Verification items for the finished model (mm, model axes). A direction names the side the tool comes from. Coordinates: 2 decimals unless noted, no trailing zeros. Order: outer loops, then holes, each group sorted by start corner. A loop starts at its lowest first (then second) coordinate and runs counter-clockwise, first axis right, second up. Notation, with made-up numbers: M 13,86.25 L 36,86.25 A31 ccw 36,112.25 Z; hole C 87.5,51 d7. An arc over 180 degrees is marked long. Use one line per item in the form item = value. Start each with the question number.
```python
from build123d import *

# Parameters (mm, degrees)
SKETCH1_R        = 3.175
EXTRUSION1_DEPTH = 6.35


with BuildPart() as part:
    # Sketch1 → Extrusion1 (new body)
    with BuildSketch(Plane.XY):
        with BuildLine():
            Line((-76.2, -6.35), (0, -6.35))
            ThreePointArc((0, -6.35), (6.35, 0), (0, 6.35))
            Line((0, 6.35), (-76.2, 6.35))
            ThreePointArc((-76.2, 6.35), (-82.55, 0), (-76.2, -6.35))
        make_face()
        with Locations((-76.2, 0)):
            Circle(SKETCH1_R, mode=Mode.SUBTRACT)
        with BuildLine():
            ThreePointArc((2.004434618, -2.462288948), (3.126764616, -0.551332964), (2.725704838, 1.62823774))
            Line((2.725704838, 1.62823774), (3.671276413, 2.755126062))
            Line((3.671276413, 2.755126062), (2.87351773, 3.424525079))
            Line((2.87351773, 3.424525079), (2.075759047, 4.093924095))
            Line((2.075759047, 4.093924095), (1.130187472, 2.967035773))
            ThreePointArc((1.130187472, 2.967035773), (-1.085913955, 2.983524071), (-2.772947665, 1.546410763))
            Line((-2.772947665, 1.546410763), (-4.221647367, 1.801855607))
            Line((-4.221647367, 1.801855607), (-4.402484579, 0.776276813))
            Line((-4.402484579, 0.776276813), (-4.583321791, -0.249301981))
            Line((-4.583321791, -0.249301981), (-3.134622089, -0.504746825))
            ThreePointArc((-3.134622089, -0.504746825), (-2.040850661, -2.432191107), (0.047242827, -3.174648503))
            Line((0.047242827, -3.174648503), (0.550370953, -4.556981669))
            Line((0.550370953, -4.556981669), (1.528966849, -4.200801892))
            Line((1.528966849, -4.200801892), (2.507562744, -3.844622115))
            Line((2.507562744, -3.844622115), (2.004434618, -2.462288948))
        make_face(mode=Mode.SUBTRACT)
    extrude(amount=EXTRUSION1_DEPTH)


solid = part.part
```
1. Material ranges on line 1 along X through (y, z) = (-2.75, 5.5); line 2 along Y through (x, z) = (-76.2, 4.25) (3 decimals); line 3 along X through (y, z) = (2, 4), recorded low to high.
2. Release check for a two-part mould opening along X. For faces 1 (the cylindrical face through (-82.55, 0.14, 3.13)), 2 (the flat face through (0.295, -3.856, 3.131)), 3 (the cylindrical face through (6.35, -0.14, 3.13)) record: pulls with the +X half, pulls with the -X half, needs draft (parallel to the pull), parting line crosses it, or undercut.
3. Depth check by flat-ended pin: P1, Ø1.5, axis at y = -2.5, z = 5, coming from the -X side; P2, Ø3, axis at y = -3, z = 2, coming from the +X side. Enter the tip coordinate at first touch or a pass-through.
4. Tool access check on faces 4 (the flat face through (-4.4, 0.8, 3.1)), 5 (the flat face through (-39, 0, 6.35)). Record the directions out of +Z, -Z, +X, -X, +Y, -Y that give a thin tool (end or side, any length) a straight path to the whole face; none if there is none.
5. Cross-section at A-A on y = -1.5. Enter the section's corners in (x, z).
6. Cross-section at B-B on z = 3.5. Enter the section's corners in (x, y) (3 decimals), and give its area (3 significant figures).
Final values:
q1.line_1 = -81.92 to -77.79, -74.61 to -1.59, 2.11 to 5.72
q1.line_2 = -6.35 to -3.175, 3.175 to 6.35
q1.line_3 = -82.23 to -78.67, -73.73 to -2.47, 3.04 to 6.03
q2.face_1 = pulls with the -X half
q2.face_2 = undercut
q2.face_3 = pulls with the +X half
q3.P1 = -82.3
q3.P2 = 6.17
q4.face_4 = +Z, -Z
q4.face_5 = +Z, +X, -X, +Y, -Y
q5.outline = M -82.37,0 L -79,0 L -79,6.35 L -82.37,6.35 Z; M -73.4,0 L -2.8,0 L -2.8,6.35 L -73.4,6.35 Z; M 2.8,0 L 6.17,0 L 6.17,6.35 L 2.8,6.35 Z
q6.outline = M -76.2,-6.35 L 0,-6.35 A6.35 ccw 0,6.35 L -76.2,6.35 A6.35 ccw Z; hole C -76.2,0 d6.35; hole M -4.583,-0.249 L -3.135,-0.505 A3.175 ccw 0.047,-3.175 L 0.55,-4.557 L 2.508,-3.845 L 2.004,-2.462 A3.175 ccw 2.726,1.628 L 3.671,2.755 L 2.076,4.094 L 1.13,2.967 A3.175 ccw -2.773,1.546 L -4.222,1.802 Z
q6.area = 1,020 mm2
